Source: CAD feature listing. Evaluate the final solid. Frame: model axes, mm. Coordinates: 2 decimals unless noted, no trailing zeros. Loops run counter-clockwise (first coordinate to the right, second up) from the corner with the lowest first, then second, coordinate; pieces in that order, holes last. Notation, with made-up numbers: (31, 43) -> (70, 43) arc R18 cw to (70, 69) -> close; hole circle Ø8 at (-8.5, 70). An arc over 180 degrees is marked (long way). Answer as CSV lines item,"result".
Autodesk Inventor part; units mm, degrees
ref_plane "YZ Plane" through (0, 0, 0) normal (1, 0, 0) x (0, 1, 0)
ref_plane "XZ Plane" through (0, 0, 0) normal (0, 1, 0) x (-1, 0, 0)
ref_plane "XY Plane" through (0, 0, 0) normal (0, 0, 1) x (1, 0, 0)
sketch "Sketch1" plane through (0, 0, 0) normal (0, 0, 1) x (1, 0, 0)
  line L0 (-55, 17.5) -> (-55, -17.5)
  line L1 (-55, 17.5) -> (55, 17.5)
  line L2 (55, 17.5) -> (55, -17.5)
  line L3 (55, -17.5) -> (-55, -17.5)
  point P0 (0, 0)
  point P1 (-55, 0)
  dimension "d0" = 35
  dimension "d1" = 55
  dimension "d2" = 110
  dimension "d3" = 35
extrude "Extrusion1" add sketch "Sketch1" against normal blind 3
sketch "Sketch2" plane through (0, 0, 0) normal (0, 0, 1) x (1, 0, 0)
  circle A0 centre (40, 0) radius 12.5
  circle A1 centre (-40, 0) radius 12.5
  point P0 (0, 0)
  dimension "d6" = 25
  dimension "d7" = 40
  dimension "d8" = 25
  dimension "d9" = 40
extrude "Extrusion2" cut sketch "Sketch2" against normal through all
properties part number "Elasma_diskou2"
(1) Cut plane C-C (z = -1.05). Return the cut outline in (x, y).
Computed values:
outline,"(-55, -17.5) -> (55, -17.5) -> (55, 17.5) -> (-55, 17.5) -> close; hole circle Ø25 at (-40, 0); hole circle Ø25 at (40, 0)"
(2) Cut plane B-B (y = 0). Return the cut outline in (x, z), then the cut area to 3 significant figures.
Computed values:
outline,"(-55, -3) -> (-52.5, -3) -> (-52.5, 0) -> (-55, 0) -> close; (-27.5, -3) -> (27.5, -3) -> (27.5, 0) -> (-27.5, 0) -> close; (52.5, -3) -> (55, -3) -> (55, 0) -> (52.5, 0) -> close"
area,"180 mm^2"
(3) Pin query (flat end, axial travel): pin 1 Ø4 at (x, y) = (31, 0.5) entering from +Z; pin 2 Ø6 at (x, y) = (-20.5, 6.5) entering from +Z. Return the tip coordinate at first contact, or that it passes through.
Computed values:
pin 1,"through"
pin 2,"z = 0"
(4) Draft query along X for faces 1 (the flat face through (-1, 0, 0)), 2 (the flat face through (-55, 0, -1)), 3 (the cylindrical face through (-49.92, -7.606, -1.479)). Return one class per face: released by +X, released by -X, zero draft, split by the parting line, or undercut.
Computed values:
face 1,"zero draft"
face 2,"released by -X"
face 3,"undercut"
(5) Cut plane D-D (y = 10). Return the cut outline in (x, z).
Computed values:
outline,"(-55, -3) -> (-47.5, -3) -> (-47.5, 0) -> (-55, 0) -> close; (-32.5, -3) -> (32.5, -3) -> (32.5, 0) -> (-32.5, 0) -> close; (47.5, -3) -> (55, -3) -> (55, 0) -> (47.5, 0) -> close"
(6) Cut plane A-A (x = 40). Return the cut outline in (y, z), then the cut area to 3 significant figures.
Computed values:
outline,"(-17.5, -3) -> (-12.5, -3) -> (-12.5, 0) -> (-17.5, 0) -> close; (12.5, -3) -> (17.5, -3) -> (17.5, 0) -> (12.5, 0) -> close"
area,"30.0 mm^2"
(7) Material intervals for L1, parallel to X at y = 11.5, z = -1; L2, parallel to X at y = 10.5, z = -2.8; L3, parallel to Y at x = -40, z = -2.25, sorted ascending. Write a range as [from, to].
Computed values:
L1,"[-55, -44.9], [-35.1, 35.1], [44.9, 55]"
L2,"[-55, -46.78], [-33.22, 33.22], [46.78, 55]"
L3,"[-17.5, -12.5], [12.5, 17.5]"
